from build123d import *

# Parameters (mm, degrees)
SKETCH_1_R          = 7.9
SKETCH_1_R_2        = 5
EXTRUDE_1_DEPTH     = 8
CUT_EXTRUDE_1_DEPTH = 4.5
SKETCH_3_R          = 15
CUT_EXTRUDE_2_DEPTH = 9
FILLET_1_R          = 20


with BuildPart() as part:
    # Эскиз1 → Бобышка-Вытянуть1 (new body)
    with BuildSketch(Plane.XY):
        with BuildLine():
            Line((-21.377154159, 5.197814933), (-52.216888254, -121.637356848))
            ThreePointArc((-52.216888254, -121.637356848), (-45.327959859, -133.591800823), (-33.055555556, -127.286710991))
            ThreePointArc((-33.055555556, -127.286710991), (0, -103.790199458), (33.055555556, -127.286710991))
            ThreePointArc((33.055555556, -127.286710991), (45.327959859, -133.591800823), (52.216888254, -121.637356848))
            Line((52.216888254, -121.637356848), (21.377154159, 5.197814933))
            ThreePointArc((21.377154159, 5.197814933), (0, 22), (-21.377154159, 5.197814933))
        make_face()
        Circle(SKETCH_1_R, mode=Mode.SUBTRACT)
        with Locations((-42.5, -124)):
            Circle(SKETCH_1_R_2, mode=Mode.SUBTRACT)
        with Locations((42.5, -124)):
            Circle(SKETCH_1_R_2, mode=Mode.SUBTRACT)
    extrude(amount=EXTRUDE_1_DEPTH)

    # Эскиз2 → Вырез-Вытянуть1 (cut)
    with BuildSketch(Plane.XY.offset(8)):
        with BuildLine():
            Line((4.5, -34.3), (-4.5, -34.3))
            ThreePointArc((-4.5, -34.3), (-11.923093689, -29.282897935), (-10.035582708, -20.524420022))
            ThreePointArc((-10.035582708, -20.524420022), (-8.5923829, -18.459875841), (-8.05, -16))
            Line((-8.05, -16), (-8.05, -15))
            ThreePointArc((-8.05, -15), (0, -6.95), (8.05, -15))
            Line((8.05, -15), (8.05, -16))
            ThreePointArc((8.05, -16), (8.5923829, -18.459875841), (10.035582708, -20.524420022))
            ThreePointArc((10.035582708, -20.524420022), (11.923093689, -29.282897935), (4.5, -34.3))
        make_face()
    extrude(amount=-CUT_EXTRUDE_1_DEPTH, mode=Mode.SUBTRACT)

    # Эскиз3 → Вырез-Вытянуть2 (cut, through all)
    with BuildSketch(Plane.XY.offset(8)):
        with Locations((-38, -56.391488719)):
            Circle(SKETCH_3_R)
        with Locations((38, -56.391488719)):
            Circle(SKETCH_3_R)
    extrude(amount=-CUT_EXTRUDE_2_DEPTH, mode=Mode.SUBTRACT)

    # Скругление1
    fillet_1_edges = [part.edges().sort_by_distance(p)[0] for p in [
        (-39.968167407, -71.261805362, 4),
        (-32.920720313, -42.277633191, 4),
        (32.920720313, -42.277633191, 4),
        (39.968167407, -71.261805362, 4),
    ]]
    fillet(fillet_1_edges, radius=FILLET_1_R)


solid = part.part
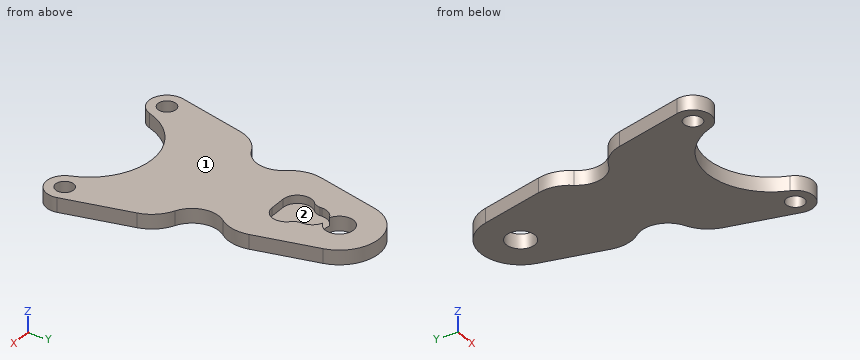
Work out the finished part from the listing and answer in its coordinate system (mm). Face numbers are marked on the shaded views. Give positions to 0.01 mm unless a question says otherwise; leave off trailing zeros. Write each loop counter-clockwise with the first axis right and the second up, starting at its lowest first coordinate (ties: lowest second). Pieces come first, ordered by that corner, then holes. Notation, with made-up numbers: M 50.25,-30.75 L 100.25,-30.75 A10 ccw 100.25,-13.75 Z; hole C -6.5,66 d10. An arc over 180 degrees is marked long. Answer as CSV lines item,"result".
Q1. A cutting plane is placed at D-D on y = -23. Write down the section's boundary in (x, z).
A:
outline,"M -28.23,0 L 28.23,0 L 28.23,8 L 11.79,8 L 11.79,3.5 L -11.79,3.5 L -11.79,8 L -28.23,8 Z"
Q2. The mould has two halves that part along Y. Classify the marked faces 1 and 2: +Y half, -Y half, draft (parallel to the pull), parting line (faces both ways), or undercut.
A:
face 1,"draft"
face 2,"undercut"
Q3. A cutting plane is placed at A-A on x = 0. Write down the section's boundary in (y, z), plus the area to 3 significant figures.
A:
outline,"M -103.79,0 L -7.9,0 L -7.9,3.5 L -34.3,3.5 L -34.3,8 L -103.79,8 Z; M 7.9,0 L 22,0 L 22,8 L 7.9,8 Z"
area,"761 mm²"
Q4. Find the intervals of material crossed by probe 1 along X at (y, z) = (-124.5, 6.5); probe 2 along Z at (x, y) = (2.5, -13.5); probe 3 along Y at (x, z) = (38.5, 0.5), in increasing order. Write a range as [from, to].
A:
probe 1,"x = [-52.49, -47.47], [-37.53, -31.95], [31.95, 37.53], [47.47, 52.49]"
probe 2,"z = [0, 3.5]"
probe 3,"y = [-133.17, -127], [-121, -75.01]"
Q5. A cutting plane is placed at C-C on y = -124. Write down the section's boundary in (x, z), plus the area to 3 significant figures.
A:
outline,"M -52.5,0 L -47.5,0 L -47.5,8 L -52.5,8 Z; M -37.5,0 L -31.72,0 L -31.72,8 L -37.5,8 Z; M 31.72,0 L 37.5,0 L 37.5,8 L 31.72,8 Z; M 47.5,0 L 52.5,0 L 52.5,8 L 47.5,8 Z"
area,"172 mm²"
Q6. Given P1, Ø4, axis at y = -36.5, z = 3.5, coming from the +X side; P2, Ø0.8, axis at y = -15.5, z = 6, coming from the +X side; P3, Ø10, axis at x = 31.5, y = 1.5, coming from the +Z side; P4, Ø4, axis at y = -14, z = 3, coming from the -X side, each flat-ended and moving along its own axis, determine where each tip first touches the part or whether it passes through.
A:
P1,"stops at x = 30.5"
P2,"stops at x = 26.51"
P3,"passes through"
P4,"stops at x = -26.53"
Q7. A cutting plane is placed at B-B on z = 5. Write down the section's boundary in (x, y), plus the area to 3 significant figures.
A:
outline,"M -52.22,-121.64 A10 ccw -33.06,-127.29 A35 cw 33.06,-127.29 A10 ccw 52.22,-121.64 L 42.95,-83.53 A20 ccw 31.79,-70.05 A15 cw 26.22,-47.11 A20 ccw 29.94,-30.01 L 21.38,5.2 A22 ccw -21.38,5.2 L -29.94,-30.01 A20 ccw -26.22,-47.11 A15 cw -31.79,-70.05 A20 ccw -42.95,-83.53 Z; hole C -42.5,-124 d10; hole M -10.04,-20.52 A8 ccw -4.5,-34.3 L 4.5,-34.3 A8 ccw 10.04,-20.52 A6.45 cw 8.05,-16 L 8.05,-15 A8.05 ccw 2.71,-7.42 A7.9 ccw long -2.71,-7.42 A8.05 ccw -8.05,-15 L -8.05,-16 A6.45 cw Z; hole C 42.5,-124 d10"
area,"7,960 mm²"
